The listing builds one solid part. Answer for the finished solid, in the listing's coordinates (mm). Give positions to 0.01 mm unless a question says otherwise; leave off trailing zeros. Write each loop counter-clockwise with the first axis right and the second up, starting at its lowest first coordinate (ties: lowest second). Pieces come first, ordered by that corner, then holes. Notation, with made-up numbers: (-18.75, 14.5) -> (18.25, 14.5) arc R12 cw to (18.25, 20.5) -> close; hole circle Ø8 at (-3.5, -15). An arc over 180 degrees is marked (long way). Use CSV: the item, a comma, the result in double quotes. Start each with the question number.
from build123d import *

# Parameters (mm, degrees)
SKETCH1_W                                        = 254
SKETCH1_H                                        = 254
BOSS_EXTRUDE1_DEPTH                              = 12.7
SKETCH2_W                                        = 203.2
SKETCH2_H                                        = 114.3
CUT_EXTRUDE1_DEPTH                               = 181.05357536
SKETCH11_W                                       = 203.2
SKETCH11_H                                       = 114.3
BOSS_EXTRUDE2_DEPTH                              = 12.7
SKETCH13_R                                       = 5.3578125
SKETCH13_R_2                                     = 6.4897
CUT_EXTRUDE8_DEPTH                               = 181.05357536
SKETCH14_R                                       = 3.1623
CUT_EXTRUDE9_DEPTH                               = 181.05357536
F_10_32_TAPPED_HOLE2_D                           = 4.0386
F_10_32_TAPPED_HOLE2_CSINK_D                     = 6.096
F_10_32_TAPPED_HOLE2_CSINK_ANGLE                 = 90
MIRROR2_COPY_1_D                                 = 4.0386
MIRROR2_COPY_1_CSINK_D                           = 6.096
MIRROR2_COPY_1_CSINK_ANGLE                       = 90
CSK_FOR_1_4_FLAT_HEAD_MACHINE_SCREW1_D           = 6.7564
CSK_FOR_1_4_FLAT_HEAD_MACHINE_SCREW1_CSINK_D     = 12.8778
CSK_FOR_1_4_FLAT_HEAD_MACHINE_SCREW1_CSINK_ANGLE = 82


with BuildPart() as part:
    # Sketch1 → Boss-Extrude1 (new body)
    with BuildSketch(Plane(origin=(0, 0, 0), x_dir=(1, 0, 0), z_dir=(0, 1, 0))):
        Rectangle(SKETCH1_W, SKETCH1_H)
    extrude(amount=BOSS_EXTRUDE1_DEPTH)

    # Sketch2 → Cut-Extrude1 (cut, through all)
    with BuildSketch(Plane(origin=(0, 12.7, 0), x_dir=(1, 0, 0), z_dir=(0, 1, 0))):
        with Locations((0, -69.85)):
            Rectangle(SKETCH2_W, SKETCH2_H)
        with Locations((0, 69.85)):
            Rectangle(SKETCH2_W, SKETCH2_H)
    extrude(amount=-CUT_EXTRUDE1_DEPTH, mode=Mode.SUBTRACT)

    # Sketch11 → Boss-Extrude2 (add)
    with BuildSketch(Plane(origin=(0, 12.7, 0), x_dir=(1, 0, 0), z_dir=(0, 1, 0))):
        with Locations((0, 69.85)):
            Rectangle(SKETCH11_W, SKETCH11_H)
        with Locations((0, -69.85)):
            Rectangle(SKETCH11_W, SKETCH11_H)
    extrude(amount=-BOSS_EXTRUDE2_DEPTH)

    # Sketch13 → Cut-Extrude8 (cut, through all)
    with BuildSketch(Plane(origin=(0, 12.7, 0), x_dir=(1, 0, 0), z_dir=(0, 1, 0))):
        with Locations(Location((86.819046868, -50.12500008, 0), (0, 0, 270))):
            Circle(SKETCH13_R)
        with Locations(Location((65.16841174, -37.625000061, 0), (0, 0, 270))):
            Circle(SKETCH13_R_2)
    extrude(amount=-CUT_EXTRUDE8_DEPTH, mode=Mode.SUBTRACT)

    # Sketch14 → Cut-Extrude9 (cut, through all)
    with BuildSketch(Plane(origin=(0, 12.7, 0), x_dir=(1, 0, 0), z_dir=(0, 1, 0))):
        with Locations(Location((77.237896866, -66.720038678, 0), (0, 0, 270))):
            Circle(SKETCH14_R)
    extrude(amount=-CUT_EXTRUDE9_DEPTH, mode=Mode.SUBTRACT)

    # #10-32 Tapped Hole2 (through all)
    with Locations(Plane(origin=(0, 12.7, 0), x_dir=(1, 0, 0), z_dir=(0, 1, 0))):
        with Locations((-114.3, -25.3365), (-114.3, -43.2435), (-114.3, -71.0565), (-114.3, -88.9635), (-88.9635, -114.3), (-71.0565, -114.3)):
            f_10_32_tapped_hole2 = CounterSinkHole(F_10_32_TAPPED_HOLE2_D / 2, F_10_32_TAPPED_HOLE2_CSINK_D / 2, counter_sink_angle=F_10_32_TAPPED_HOLE2_CSINK_ANGLE)

    # Mirror1: #10-32 Tapped Hole2 across plane
    add(f_10_32_tapped_hole2.mirror(Plane.XY), mode=Mode.SUBTRACT)

    # Mirror2: #10-32 Tapped Hole2 across plane
    add(f_10_32_tapped_hole2.mirror(Plane(origin=(0, 0, 0), x_dir=(0, 0, 1), z_dir=(1, 0, 0))), mode=Mode.SUBTRACT)

    # Mirror2 copy 1 (through all)
    with Locations(Plane(origin=(0, 12.7, 0), x_dir=(-1, 0, 0), z_dir=(0, 1, 0))):
        with Locations((-114.3, -25.3365), (-114.3, -43.2435), (-114.3, -71.0565), (-114.3, -88.9635), (-88.9635, -114.3), (-71.0565, -114.3)):
            CounterSinkHole(MIRROR2_COPY_1_D / 2, MIRROR2_COPY_1_CSINK_D / 2, counter_sink_angle=MIRROR2_COPY_1_CSINK_ANGLE)

    # CSK for 1/4 Flat Head Machine Screw1 (through all)
    with Locations(Plane(origin=(0, 12.7, 0), x_dir=(1, 0, 0), z_dir=(0, 1, 0))):
        with Locations((-114.3, 0), (-114.3, 114.3), (-114.3, -114.3)):
            csk_for_1_4_flat_head_machine_screw1 = CounterSinkHole(CSK_FOR_1_4_FLAT_HEAD_MACHINE_SCREW1_D / 2, CSK_FOR_1_4_FLAT_HEAD_MACHINE_SCREW1_CSINK_D / 2, counter_sink_angle=CSK_FOR_1_4_FLAT_HEAD_MACHINE_SCREW1_CSINK_ANGLE)

    # Mirror3: CSK for 1/4 Flat Head Machine Screw1 across plane
    add(csk_for_1_4_flat_head_machine_screw1.mirror(Plane(origin=(0, 0, 0), x_dir=(0, 0, 1), z_dir=(1, 0, 0))), mode=Mode.SUBTRACT)


solid = part.part
Q1. Straight lines are drawn through the part: L1, parallel to Z at x = -72, y = 7.75; L2, parallel to Z at x = 77.5, y = 9.25; L3, parallel to X at y = 6, z = 69. For each, find the intervals that lie inside material, in ascending order.
Q2. Section A-A on z = 0 is taken. Give the vertices of the cut face in (x, y).
Q3. Flat-ended cylindrical pins translate along their axes: pin 1 Ø5.5 at (x, z) = (-114.3, 114.3) entering from -Y; pin 2 Ø4.5 at (x, z) = (88.96, 114.3) entering from +Y; pin 3 Ø5.5 at (x, z) = (-71.06, 114.3) entering from +Y. Find the tip coordinate at first contact, or state that the pin passes through.
Q4. The mould has two halves that part along X. Classify faces 1 (the face through (-127, 6, 2)), 2 (the face through (117.522, 4.525, 113.285)), 3 (the face through (-2, 6, -127)): +X half, -X half, draft (parallel to the pull), parting line (faces both ways), or undercut.
Output:
1,L1,"-127 to -116.09, -112.51 to 112.51, 116.09 to 127"
1,L2,"-127 to 63.57, 69.87 to 127"
1,L3,"-127 to 75.05, 79.43 to 127"
2,outline,"(-127, 0) -> (-117.68, 0) -> (-117.68, 9.18) -> (-120.74, 12.7) -> (-127, 12.7) -> close; (-110.92, 0) -> (110.92, 0) -> (110.92, 9.18) -> (107.86, 12.7) -> (-107.86, 12.7) -> (-110.92, 9.18) -> close; (117.68, 0) -> (127, 0) -> (127, 12.7) -> (120.74, 12.7) -> (117.68, 9.18) -> close"
3,pin 1,"through"
3,pin 2,"y = 11.91"
3,pin 3,"y = 12.41"
4,face 1,"-X half"
4,face 2,"undercut"
4,face 3,"draft"
